Model file for the job. Use its own axes, mm. A direction names the side the tool comes from. Coordinates: 2 decimals unless noted, no trailing zeros. Return JSON: item names as keys, results as strings. Group by question number.
1) Cut at B-B (y = -1.75). State how many separate pieces and enclosed holes the cut face has, and give its area (3 significant figures).
2) Flat gauge pins, fed straight in: pin 1 (10 mm diameter, centred on y = 0, z = 6.5, fed in from -X); pin 2 (4 mm diameter, centred on x = 26.99, z = 46.74, fed in from +Y); pin 3 (2 mm diameter, centred on y = 15, z = 23, fed in from +X) (3 decimals); pin 4 (3 mm diameter, centred on x = 53.975, z = 0, fed in from -Y). Where does each tip first touch, or does it go through?
3) Which spindle directions (+Z, -Z, +X, -X, +Y, -Y) get a long thin tool onto all of the face, cutting with end or side? Do faces 1 (the cylindrical face through (-11.012, 16.492, -49.592)), 2 (the flat face through (-27, 15.24, -42)), 3 (the cylindrical face through (52.224, -3.091, 0.077)). Say none if no direction does.
4) Probe line 1 (X direction, y = -1.5, z = 47); line 2 (Z direction, x = 26, y = -1.75); line 3 (X direction, y = 11.25, z = 0). List the from-to ranges inside material, lowest first.
5) Pull direction Z, two halves, no side cores. Call faces 4 (the cylindrical face through (26.8, -3.1, -45)), 5 (the flat face through (-27, 12.065, -42)), 6 (the cylindrical face through (46.94, 13.67, -14.78)): +Z half, -Z half, draft (parallel to the pull), parting line (faces both ways), or undercut.
Autodesk Inventor part; units mm, degrees
ref_plane "YZ Plane" through (0, 0, 0) normal (1, 0, 0) x (0, 1, 0)
ref_plane "XZ Plane" through (0, 0, 0) normal (0, 1, 0) x (-1, 0, 0)
ref_plane "XY Plane" through (0, 0, 0) normal (0, 0, 1) x (1, 0, 0)
sketch "Sketch1" plane through (0, 0, 0) normal (0, 1, 0) x (-1, 0, 0)
  circle A0 centre (0, 0) radius 50.8
  dimension "d0" = 101.6
extrude "Extrusion1" add sketch "Sketch1" along normal blind 7.62
sketch "Sketch2" plane through (0, 7.62, 0) normal (0, 1, 0) x (1, 0, 0)
  circle A0 centre (0, 0) radius 49.2125
  circle A1 centre (0, 0) radius 50.8
  dimension "d3" = 98.425
extrude "Extrusion2" cut sketch "Sketch2" against normal blind 3.175
sketch "Sketch3" plane through (0, 7.62, 0) normal (0, 1, 0) x (1, 0, 0)
  circle A0 centre (0, 0) radius 50.9584
extrude "Extrusion3" add sketch "Sketch3" along normal blind 7.62
sketch "Sketch4" plane through (0, 15.24, 0) normal (0, 1, 0) x (1, 0, 0)
  point P0 (0, 0)
sketch "Sketch5" plane through (0, 15.24, 0) normal (0, 1, 0) x (1, 0, 0)
  circle A0 centre (0, 0) radius 49.2125
  circle A1 centre (0, 0) radius 50.9584
  dimension "d8" = 98.425
extrude "Extrusion4" cut sketch "Sketch5" against normal blind 3.175
sketch "Sketch6" plane through (0, 15.24, 0) normal (0, 1, 0) x (1, 0, 0)
  circle A0 centre (0, 0) radius 50.8
  dimension "d11" = 101.6
extrude "Extrusion5" add sketch "Sketch6" along normal blind 5.08
sketch "Sketch7" plane through (0, 0, 0) normal (0, -1, 0) x (1, 0, 0)
  circle A0 centre (0, 0) radius 57.15
  dimension "d14" = 114.3
extrude "Extrusion6" add sketch "Sketch7" along normal blind 6.096
chamfer "Chamfer1" distance 2.54 angle 45 1 edges at (-50.8, 20.32, 0)
sketch "Sketch8" plane through (0, -6.096, 0) normal (0, -1, 0) x (1, 0, 0)
  circle A0 centre (0, 0) radius 50.8
  circle A1 centre (53.975, 0) radius 1.7526
  circle A2 centre (26.9875, 46.7437) radius 1.7526
  circle A3 centre (-26.9875, 46.7437) radius 1.7526
  circle A4 centre (-53.975, 0) radius 1.7526
  circle A5 centre (-26.9875, -46.7437) radius 1.7526
  circle A6 centre (26.9875, -46.7437) radius 1.7526
  dimension "d20" = 3.5052
  dimension "d21" = 53.975
  dimension "d24" = 360
extrude "Extrusion7" cut sketch "Sketch8" against normal blind 6.096 contours A1 | A2 | A3 | A4 | A5 | A6
sketch "Sketch9" plane through (0, -6.096, 0) normal (0, -1, 0) x (1, 0, 0)
  circle A0 centre (0, 0) radius 12.7
  circle A1 centre (0, 0) radius 1.27
  dimension "d28" = 25.4
  dimension "d29" = 2.54
extrude "Extrusion8" cut sketch "Sketch9" against normal blind 127 contours A1
sketch "Sketch10" plane through (0, -6.096, 0) normal (0, -1, 0) x (1, 0, 0)
  circle A0 centre (0, 0) radius 1.27
  circle A1 centre (0, 0) radius 38.1
  dimension "d33" = 76.2
extrude "Extrusion9" cut sketch "Sketch10" against normal blind 9.525
sketch "Sketch11" plane through (0, 3.429, 0) normal (0, -1, 0) x (1, 0, 0)
  circle A0 centre (0, 0) radius 12.7
  circle A1 centre (0, 0) radius 1.27
  dimension "d36" = 25.4
extrude "Extrusion10" add sketch "Sketch11" along normal blind 9.525
sketch "Sketch12" plane through (0, 20.32, 0) normal (0, 1, 0) x (1, 0, 0)
  circle A0 centre (0, 0) radius 1.27
  circle A1 centre (0, 0) radius 38.1
extrude "Extrusion11" cut sketch "Sketch12" against normal blind 508
sketch "Sketch13" plane through (0, -6.096, 0) normal (0, -1, 0) x (1, 0, 0)
  point P0 (0, 0)
properties part number "O ring Dome 2"
Answers below:
{
 "1": {"separate pieces": "1", "enclosed holes": "7", "area": "5,640 mm^2"},
 "2": {"pin 1": "stops at x = -57.13", "pin 2": "stops at y = 0", "pin 3": "stops at x = 45.775", "pin 4": "passes through"},
 "3": {"face 1": "+Y", "face 2": "none", "face 3": "+Y, -Y"},
 "4": {"line 1": "x = -32.51 to -28.72, -25.25 to 25.25, 28.72 to 32.51", "line 2": "z = -50.89 to -48.19, -45.3 to -27.85, 27.85 to 45.3, 48.19 to 50.89", "line 3": "x = -50.96 to -38.1, 38.1 to 50.96"},
 "5": {"face 4": "undercut", "face 5": "draft", "face 6": "parting line"}
}
